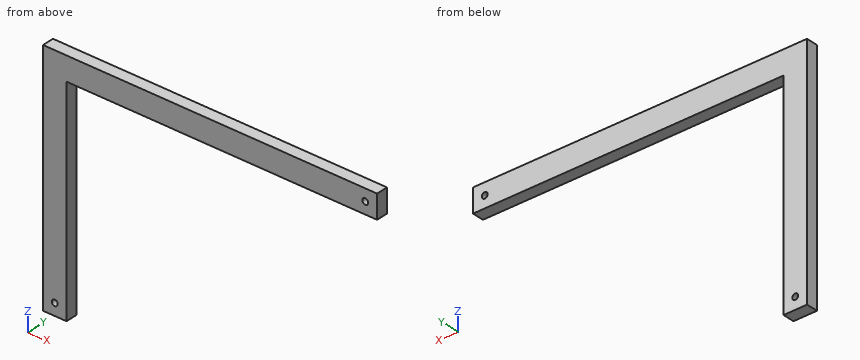
Autodesk Inventor part; units mm, degrees
ref_plane "YZ Plane" through (0, 0, 0) normal (1, 0, 0) x (0, 1, 0)
ref_plane "XZ Plane" through (0, 0, 0) normal (0, 1, 0) x (-1, 0, 0)
ref_plane "XY Plane" through (0, 0, 0) normal (0, 0, 1) x (1, 0, 0)
sketch "Sketch7" plane through (0, 0, 0) normal (1, 0, 0) x (0, 1, 0)
  line L0 (6.35, 12.7) -> (-6.35, 12.7)
  line L1 (-6.35, 12.7) -> (-6.35, -12.7)
  line L2 (-6.35, -12.7) -> (6.35, -12.7)
  line L3 (6.35, -12.7) -> (6.35, 12.7)
  line L4 (6.35, 12.7) -> (-6.35, -12.7) construction
  line L5 (-6.35, 12.7) -> (6.35, -12.7) construction
  point P0 (0, 0)
  dimension "d30" = 12.7
  dimension "d31" = 25.4
sketch "Sketch9" plane through (0, 0, 0) normal (0, 1, 0) x (-1, 0, 0)
  line L0 (0, 0) -> (348.0816, 0)
  line L1 (348.0816, 0) -> (348.0816, -244.729)
  dimension "d34" = 244.729
  dimension "d35" = 348.0816
sweep "Sweep2" add profiles "Sketch7" path "Sketch9"
sketch "Sketch10" plane through (0, 6.35, 12.7) normal (0, 1, 0) x (1, 0, 0)
  line L0 (0, 0) -> (0, 25.4)
  line L1 (0, 25.4) -> (-335.3816, 25.4)
  line L2 (0, 0) -> (-25.4, 0)
  line L3 (-25.4, 0) -> (-25.4, 25.4)
  line L4 (-25.4, 25.4) -> (0, 25.4)
  line L5 (0, 25.4) -> (0, 0)
  circle A0 centre (-12.7, 12.7) radius 3.175
  line L6 (-335.3816, 257.429) -> (-360.7816, 257.429)
  line L7 (-360.7816, 0) -> (-360.7816, 257.429)
  line L8 (-335.3816, 257.429) -> (-360.7816, 257.429)
  line L9 (-360.7816, 257.429) -> (-360.7816, 232.029)
  line L10 (-360.7816, 232.029) -> (-335.3816, 232.029)
  line L11 (-335.3816, 232.029) -> (-335.3816, 257.429)
  circle A1 centre (-348.0816, 244.729) radius 3.175
  point P0 (0, 12.7)
  point P1 (-25.4, 12.7)
  point P2 (-12.7, 25.4)
  dimension "d38" = 25.4
  dimension "d39" = 6.35
  dimension "d40" = 12.7
  dimension "d41" = 12.7
  dimension "d42" = 25.4
  dimension "d43" = 6.35
  dimension "d44" = 12.7
  dimension "d45" = 12.7
extrude "Extrusion4" cut sketch "Sketch10" against normal blind 25.4 contours A0 | A1
properties part number "ArmRest(H)"
Source: CAD feature listing. Evaluate the final solid. Frame: model axes, mm. Round coordinates to 2 decimals unless told otherwise and drop trailing zeros. Write each loop counter-clockwise with the first axis right and the second up, starting at its lowest first coordinate (ties: lowest second). Pieces come first, ordered by that corner, then holes. Notation, with made-up numbers: M -10,2 L 4,2 A33 ccw 4,31 Z; hole C 60.5,15.5 d3. An arc over 180 degrees is marked long. Answer as a JSON object with one key per item and string values. Group by question number.
(1) Ray query, line 1 (X direction, y = 1, z = 0) (3 decimals); line 2 (Z direction, x = -12.7, y = -1) (3 decimals); line 3 (Z direction, x = -192.5, y = 0). Return the intervals inside material, ascending. Write a range as [from, to].
(2) First-contact query: pin 1 (6.5 mm diameter, centred on x = -181.5, y = 1.5, fed in from -Z); pin 2 (3 mm diameter, centred on y = -1, z = -176.5, fed in from +X); pin 3 (5 mm diameter, centred on x = -12.7, z = 0, fed in from +Y). Flat tips, straight axial feed; report the tip coordinate or a pass-through.
(3) Section query C-C on z = -119. Output: boundary loops of the cut face in (x, y), then the cut area to 3 significant figures.
(4) Section query B-B on x = -113. Output: boundary loops of the cut face in (y, z), then the cut area to 3 significant figures.
(5) Section query A-A on y = 3.25. Output: boundary loops of the cut face in (x, z) (3 decimals).
Computed values:
{
 "1": {"line 1": "[-360.782, -15.875], [-9.525, 0]", "line 2": "[-12.7, -3.175], [3.175, 12.7]", "line 3": "[-12.7, 12.7]"},
 "2": {"pin 1": "z = -12.7", "pin 2": "x = -335.38", "pin 3": "through"},
 "3": {"outline": "M -360.78,-6.35 L -335.38,-6.35 L -335.38,6.35 L -360.78,6.35 Z", "area": "323 mm^2"},
 "4": {"outline": "M -6.35,-12.7 L 6.35,-12.7 L 6.35,12.7 L -6.35,12.7 Z", "area": "323 mm^2"},
 "5": {"outline": "M -360.782,-244.729 L -335.382,-244.729 L -335.382,-12.7 L 0,-12.7 L 0,12.7 L -360.782,12.7 Z; hole C -348.082,-232.029 d6.35; hole C -12.7,0 d6.35"}
}
